```python
from build123d import *

# Parameters (mm, degrees)
SKETCH1_W            = 57.131427428
SKETCH1_H            = 41
BOSS_EXTRUDE1_DEPTH  = 2
SKETCH2_W            = 28.565713714
SKETCH2_H            = 2
BOSS_EXTRUDE2_DEPTH  = 2
CUT_EXTRUDE4_DEPTH   = 2
LPATTERN1_COUNT      = 4
LPATTERN1_PITCH      = 9.5
MIRROR2_COPY_1_DEPTH = 2
MIRROR2_COPY_2_DEPTH = 2
MIRROR2_COPY_3_DEPTH = 2
FILLET1_R            = 1
FILLET2_R            = 2


with BuildPart() as part:
    # Sketch1 → Boss-Extrude1 (new body)
    with BuildSketch(Plane(origin=(0, 0, 0), x_dir=(1, 0, 0), z_dir=(0, 1, 0))):
        with Locations((0, 20.5)):
            Rectangle(SKETCH1_W, SKETCH1_H)
    extrude(amount=BOSS_EXTRUDE1_DEPTH)

    # Sketch2 → Boss-Extrude2 (add)
    with BuildSketch(Plane.XZ):
        with Locations((-14.282856857, -1)):
            Rectangle(SKETCH2_W, SKETCH2_H)
        with Locations((14.282856857, -1)):
            Rectangle(SKETCH2_W, SKETCH2_H)
        Polygon((1.5, -20), (3.5, -20), (3.5, -6), (28.565713714, -6), (28.565713714, -4), (1.5, -4), align=None)
        Polygon((-28.565713714, -6), (-28.565713714, -4), (-1.5, -4), (-1.5, -20), (-3.5, -20), (-3.5, -6), align=None)
    extrude(amount=BOSS_EXTRUDE2_DEPTH)

    # Sketch4 → Revolve1 (revolve)
    with BuildSketch(Plane.XZ):
        with BuildLine():
            Line((-26.565713714, 0), (-28.565713714, 0))
            ThreePointArc((-28.565713714, 0), (-27.979927277, 1.414213562), (-26.565713714, 2))
            Line((-26.565713714, 2), (-26.565713714, 0))
        make_face()
    revolve1 = revolve(axis=Axis((-26.565713714, 0, 0), (0, 0, 1)))

    # Mirror1: Revolve1 across plane
    add(revolve1.mirror(Plane(origin=(0, 0, 0), x_dir=(0, 0, 1), z_dir=(1, 0, 0))))

    # Sketch7 → Cut-Extrude4 (cut)
    with BuildSketch(Plane(origin=(0, 2, 0), x_dir=(1, 0, 0), z_dir=(0, 1, 0))):
        with BuildLine():
            Line((-24.076247257, 8.949248512), (-24.606518128, 9.282743394))
            ThreePointArc((-24.606518128, 9.282743394), (-26.412219505, 9.532379514), (-25.405087398, 8.012984708))
            Line((-25.405087398, 8.012984708), (-24.129168598, 7.210541254))
            Line((-24.129168598, 7.210541254), (-23.60872049, 6.883224049))
            ThreePointArc((-23.60872049, 6.883224049), (-22.810789527, 6.765633149), (-22.185605476, 7.275207818))
            ThreePointArc((-22.185605476, 7.275207818), (-22.329575973, 10.981780083), (-25.565713714, 12.794738433))
            Line((-25.565713714, 12.794738433), (-28.565713714, 12.794738433))
            Line((-28.565713714, 12.794738433), (-28.565713714, 11.294738433))
            Line((-28.565713714, 11.294738433), (-25.565713714, 11.294738433))
            ThreePointArc((-25.565713714, 11.294738433), (-24.121260099, 10.783081105), (-23.320945498, 9.476277368))
            ThreePointArc((-23.320945498, 9.476277368), (-23.52393963, 8.962456819), (-24.076247257, 8.949248512))
        make_face()
    cut_extrude4 = extrude(amount=-CUT_EXTRUDE4_DEPTH, mode=Mode.SUBTRACT)

    # LPattern1: Cut-Extrude4 ×4
    with Locations(*[(0, 0, -i * LPATTERN1_PITCH) for i in range(1, LPATTERN1_COUNT)]):
        add(cut_extrude4, mode=Mode.SUBTRACT)

    # Mirror2: Cut-Extrude4 across plane
    add(cut_extrude4.mirror(Plane(origin=(0, 0, 0), x_dir=(0, 0, 1), z_dir=(1, 0, 0))), mode=Mode.SUBTRACT)

    # Mirror2 copy 1 sketch → Mirror2 copy 1 (cut)
    with BuildSketch(Plane(origin=(0, 2, -9.5), x_dir=(-1, 0, 0), z_dir=(0, 1, 0))):
        with BuildLine():
            Line((-24.076247257, -8.949248512), (-24.606518128, -9.282743394))
            ThreePointArc((-24.606518128, -9.282743394), (-26.412219505, -9.532379514), (-25.405087398, -8.012984708))
            Line((-25.405087398, -8.012984708), (-24.129168598, -7.210541254))
            Line((-24.129168598, -7.210541254), (-23.60872049, -6.883224049))
            ThreePointArc((-23.60872049, -6.883224049), (-22.810789527, -6.765633149), (-22.185605476, -7.275207818))
            ThreePointArc((-22.185605476, -7.275207818), (-22.329575973, -10.981780083), (-25.565713714, -12.794738433))
            Line((-25.565713714, -12.794738433), (-28.565713714, -12.794738433))
            Line((-28.565713714, -12.794738433), (-28.565713714, -11.294738433))
            Line((-28.565713714, -11.294738433), (-25.565713714, -11.294738433))
            ThreePointArc((-25.565713714, -11.294738433), (-24.121260099, -10.783081105), (-23.320945498, -9.476277368))
            ThreePointArc((-23.320945498, -9.476277368), (-23.52393963, -8.962456819), (-24.076247257, -8.949248512))
        make_face()
    extrude(amount=-MIRROR2_COPY_1_DEPTH, mode=Mode.SUBTRACT)

    # Mirror2 copy 2 sketch → Mirror2 copy 2 (cut)
    with BuildSketch(Plane(origin=(0, 2, -19), x_dir=(-1, 0, 0), z_dir=(0, 1, 0))):
        with BuildLine():
            Line((-24.076247257, -8.949248512), (-24.606518128, -9.282743394))
            ThreePointArc((-24.606518128, -9.282743394), (-26.412219505, -9.532379514), (-25.405087398, -8.012984708))
            Line((-25.405087398, -8.012984708), (-24.129168598, -7.210541254))
            Line((-24.129168598, -7.210541254), (-23.60872049, -6.883224049))
            ThreePointArc((-23.60872049, -6.883224049), (-22.810789527, -6.765633149), (-22.185605476, -7.275207818))
            ThreePointArc((-22.185605476, -7.275207818), (-22.329575973, -10.981780083), (-25.565713714, -12.794738433))
            Line((-25.565713714, -12.794738433), (-28.565713714, -12.794738433))
            Line((-28.565713714, -12.794738433), (-28.565713714, -11.294738433))
            Line((-28.565713714, -11.294738433), (-25.565713714, -11.294738433))
            ThreePointArc((-25.565713714, -11.294738433), (-24.121260099, -10.783081105), (-23.320945498, -9.476277368))
            ThreePointArc((-23.320945498, -9.476277368), (-23.52393963, -8.962456819), (-24.076247257, -8.949248512))
        make_face()
    extrude(amount=-MIRROR2_COPY_2_DEPTH, mode=Mode.SUBTRACT)

    # Mirror2 copy 3 sketch → Mirror2 copy 3 (cut)
    with BuildSketch(Plane(origin=(0, 2, -28.5), x_dir=(-1, 0, 0), z_dir=(0, 1, 0))):
        with BuildLine():
            Line((-24.076247257, -8.949248512), (-24.606518128, -9.282743394))
            ThreePointArc((-24.606518128, -9.282743394), (-26.412219505, -9.532379514), (-25.405087398, -8.012984708))
            Line((-25.405087398, -8.012984708), (-24.129168598, -7.210541254))
            Line((-24.129168598, -7.210541254), (-23.60872049, -6.883224049))
            ThreePointArc((-23.60872049, -6.883224049), (-22.810789527, -6.765633149), (-22.185605476, -7.275207818))
            ThreePointArc((-22.185605476, -7.275207818), (-22.329575973, -10.981780083), (-25.565713714, -12.794738433))
            Line((-25.565713714, -12.794738433), (-28.565713714, -12.794738433))
            Line((-28.565713714, -12.794738433), (-28.565713714, -11.294738433))
            Line((-28.565713714, -11.294738433), (-25.565713714, -11.294738433))
            ThreePointArc((-25.565713714, -11.294738433), (-24.121260099, -10.783081105), (-23.320945498, -9.476277368))
            ThreePointArc((-23.320945498, -9.476277368), (-23.52393963, -8.962456819), (-24.076247257, -8.949248512))
        make_face()
    extrude(amount=-MIRROR2_COPY_3_DEPTH, mode=Mode.SUBTRACT)

    # Fillet1
    fillet1_edges = [part.edges().sort_by_distance(p)[0] for p in [
        (1.5, -1, -4),
        (-1.5, -1, -4),
    ]]
    fillet(fillet1_edges, radius=FILLET1_R)

    # Fillet2
    fillet2_edges = [part.edges().sort_by_distance(p)[0] for p in [
        (-24.099412322, 1, -41),
        (24.099412322, 1, -41),
    ]]
    fillet(fillet2_edges, radius=FILLET2_R)


solid = part.part
```
Could you check a few things on this model? Use its own coordinates, in mm. A direction names the side the tool comes from. Give positions to 0.01 mm unless a question says otherwise; leave off trailing zeros. Write each loop counter-clockwise with the first axis right and the second up, starting at its lowest first coordinate (ties: lowest second). Pieces come first, ordered by that corner, then holes. Notation, with made-up numbers: (66, 25.25) -> (97, 25.25) arc R37 cw to (97, 62.25) -> close; hole circle Ø10 at (84, 13). An arc over 180 degrees is marked (long way). Write each question's results on one line, items separated by ' | '.
1. I want a section at B-B, the plane x = -7. Write out the boundary of the cut face in (y, z).
Check sheet entries:
outline: (-2, -6) -> (0, -6) -> (0, -41) -> (2, -41) -> (2, 0) -> (-2, 0) -> (-2, -2) -> (0, -2) -> (0, -4) -> (-2, -4) -> close
2. On a 3-axis mill with a long thin cutter (end or side, diameter ignored), from which of +Z, -Z, +X, -X, +Y, -Y can I reach the whole of each face in a straight line? I mean faces 1 (the flat face through (16, -1, -4)), 2 (the flat face through (27, 1, -11.295)), 3 (the flat face through (-1.5, -1, -12)), 4 (the flat face through (-27, 1, -12.795)), 5 (the cylindrical face through (-24.14, 1.01, -10.8)). Say none if no direction works.
Check sheet entries:
face 1: +X, -X, -Y | face 2: +X, +Y, -Y | face 3: -Z, -Y | face 4: -X, +Y, -Y | face 5: +Y, -Y
3. I want a section at A-A, the plane z = -15. Write out the boundary of the cut face in (x, y).
Check sheet entries:
outline: (-28.57, 0) -> (-3.5, 0) -> (-3.5, -2) -> (-1.5, -2) -> (-1.5, 0) -> (1.5, 0) -> (1.5, -2) -> (3.5, -2) -> (3.5, 0) -> (28.57, 0) -> (28.57, 2) -> (-28.57, 2) -> close
4. I need wall thicknesses on L1, parallel to X at y = 0.65, z = -37; L2, parallel to Z at x = 5.5, y = -0.05; L3, parallel to X at y = 1, z = -9. Which ranges of each line are inside material? Lowest first, please.
Check sheet entries:
L1: x = -28.57 to -26.43, -21.8 to 21.8, 26.43 to 28.57 | L2: z = -6 to -4, -2 to 0 | L3: x = -28.57 to -26.57, -24.16 to -23.48, -21.77 to 21.77, 23.48 to 24.16, 26.57 to 28.57
5. If we mould it in two halves opening along Z, with no side actions, what happens to faces 6 (the flat face through (28.2, 1.5, 0)), 7 (the cylindrical face through (-24.14, 1.01, -39.3)), 8 (the cylindrical face through (-26.395, 1.014, -19.059))? For each: released by +Z, released by -Z, zero draft, split by the parting line, or undercut.
Check sheet entries:
face 6: released by +Z | face 7: released by -Z | face 8: undercut
6. Will these pins go through, and if not, where does the flat tip stop? pin 1 Ø1 at (x, y) = (-27.5, 0.5) entering from -Z; pin 2 Ø1.5 at (y, z) = (-1, -30.5) entering from -X; pin 3 Ø1.5 at (x, y) = (-3.5, 0) entering from +Z; pin 4 Ø1.6 at (x, y) = (-27.5, 0.5) entering from +Z.
Check sheet entries:
pin 1: stops at z = -39.79 | pin 2: passes through | pin 3: stops at z = 0 | pin 4: stops at z = 1.98
